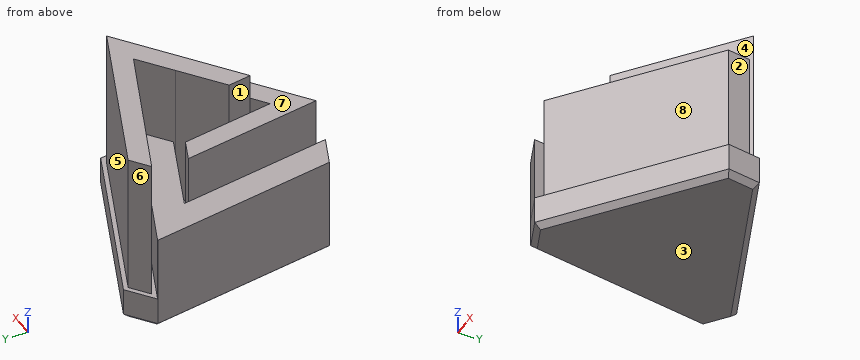
```python
from build123d import *

# Parameters (mm, degrees)
F1_DEPTH = 30
F5_DEPTH = 60
F6_DEPTH = 100
F7_DEPTH = 130
F8_SIZE  = 5


with BuildPart() as f1:
    # F0 (on Top) → F1 (new body)
    with BuildSketch(Plane.XY):
        Polygon((-39.487894, -75.850017), (94.227236, 28.575137), (90.058191, 58.284042), (-67.23421, 121.872165), (-90.878354, 103.407213), (-67.301084, -64.606063), align=None)
    extrude(amount=F1_DEPTH)

    # F2 (on face) → F5 (join)
    with BuildSketch(Plane.XY.offset(30)):
        Polygon((14.600857, 32.81471), (37.999574, 51.148787), (-90.714814, 103.534931), (-90.878354, 103.407213), (-67.301084, -64.606063), (-40.06353, -75.617306), (-59.289651, 62.461207), (-30.906815, 51.073389), align=None)
    extrude(amount=F5_DEPTH)

    # F4 (on face) → F6 (join)
    with BuildSketch(Plane.XY.offset(30)):
        Polygon((87.029812, 51.080902), (-23.003388, -34.692019), (-28.099764, 1.909229), (-34.548747, 48.224661), (-54.376458, 56.179975), (-36.972718, -68.81053), (89.945114, 30.306257), align=None)
    extrude(amount=F6_DEPTH)

    # F3 (on face) → F7 (join)
    with BuildSketch(Plane.XY.offset(30)):
        Polygon((17.067929, 29.66613), (-19.8587, 0.732249), (-16.991157, -19.861924), (81.935531, 57.253266), (-66.592344, 117.29818), (-82.807181, 104.635163), (45.895328, 52.253855), align=None)
    extrude(amount=F7_DEPTH)

    # F8
    f8_edges = [f1.edges().sort_by_distance(p)[0] for p in [
        (11.41199, 90.078103, 0),
        (92.142713, 43.429589, 0),
        (27.369671, -23.63744, 0),
        (-79.056282, 112.639689, 0),
        (-79.089719, 19.400575, 0),
        (-53.394489, -70.22804, 0),
    ]]
    chamfer(f8_edges, length=F8_SIZE)


solid = f1.part
```
Read the model definition and answer for the solid it produces. Units are mm, in the model's axes. Face numbers are marked on the shaded views. A direction names the side the tool comes from. Coordinates: 2 decimals unless noted, no trailing zeros. Write each loop counter-clockwise with the first axis right and the second up, starting at its lowest first coordinate (ties: lowest second). Pieces come first, ordered by that corner, then holes. Notation, with made-up numbers: (-4, -8.5) -> (1, -8.5) arc R23 ccw to (1, 29.5) -> close; hole circle Ø5 at (30.25, 0). An arc over 180 degrees is marked (long way). Write item = value, one per line.
(1) Which of the six approach directions +Z, -Z, +X, -X, +Y, -Y give full straight-line access (tool end or side, diameter ignored) to the marked faces 4, 5, 6, 7 and 8?
From the geometry:
face_4 = +Z
face_5 = +Z, +X, +Y
face_6 = +Z, -X, +Y
face_7 = +Z, -Y
face_8 = +Z, +X, -Y
(2) For a pull along X with two mould halves and no side action, classify the marked faces 1, 2 and 3 as +X half, -X half, draft (parallel to the pull), parting line (faces both ways), or undercut.
From the geometry:
face_1 = undercut
face_2 = +X half
face_3 = draft
(3) Section B-B on z = 48 is taken. Write down the section's boundary in (x, y), plus the area to 3 significant figures.
From the geometry:
outline = (-90.88, 103.41) -> (-67.3, -64.61) -> (-40.06, -75.62) -> (-59.29, 62.46) -> (14.6, 32.81) -> (38, 51.15) -> (-90.71, 103.53) -> close; (-82.81, 104.64) -> (45.9, 52.25) -> (-19.86, 0.73) -> (-16.99, -19.86) -> (81.94, 57.25) -> (-66.59, 117.3) -> close; (-54.38, 56.18) -> (-36.97, -68.81) -> (89.95, 30.31) -> (87.03, 51.08) -> (-23, -34.69) -> (-34.55, 48.22) -> close
area = 16,100 mm2
(4) Given pin 1 Ø1.5 at (x, z) = (49, 69) entering from -Y; pin 2 Ø6 at (y, z) = (36, 133.5) entering from -X; pin 3 Ø12 at (y, z) = (-13.5, 109.5) entering from -X, each flat-ended and moving along its own axis, determine where each tip first touches the part or whether it passes through.
From the geometry:
pin_1 = -2.26
pin_2 = 21.32
pin_3 = -45.51
(5) Section C-C on x = 2.5 is taken. Write down the section's boundary in (y, z).
From the geometry:
outline = (-43.06, 5) -> (-36.72, 0) -> (88.29, 0) -> (93.68, 5) -> (93.68, 30) -> (89.37, 30) -> (89.37, 160) -> (69.92, 160) -> (69.92, 30) -> (65.6, 30) -> (65.6, 90) -> (37.67, 90) -> (37.67, 30) -> (18.25, 30) -> (18.25, 160) -> (-4.67, 160) -> (-4.67, 30) -> (-14.81, 30) -> (-14.81, 130) -> (-37.98, 130) -> (-37.98, 30) -> (-43.06, 30) -> close
(6) Section A-A on z = 112.5 is taken. Write down the section's boundary in (x, y).
From the geometry:
outline = (-82.81, 104.64) -> (45.9, 52.25) -> (-19.86, 0.73) -> (-16.99, -19.86) -> (81.94, 57.25) -> (-66.59, 117.3) -> close; (-54.38, 56.18) -> (-36.97, -68.81) -> (89.95, 30.31) -> (87.03, 51.08) -> (-23, -34.69) -> (-34.55, 48.22) -> close
(7) Straight lines are drawn through the part: L1, parallel to X at y = 18.5, z = 111.5; L2, parallel to Y at x = 10, z = 111; L3, parallel to X at y = -18, z = 52. For each, find the intervals that lie inside material, in ascending order. Write a range as from..to.
From the geometry:
L1 = -49.13..-30.41, 2.82..32.22, 45.23..74.83
L2 = -32.13..-8.97, 1.18..24.13, 66.86..86.33
L3 = -73.84..-48.09, -44.05..-25.33, -17.25..-14.6, -1.59..28.09
(8) Section D-D on y = 98 is taken. Write down the section's boundary in (x, z).
From the geometry:
outline = (-90.12, 5) -> (-85.07, 0) -> (-21.52, 0) -> (-8.18, 5) -> (-8.18, 30) -> (-18.86, 30) -> (-18.86, 160) -> (-66.5, 160) -> (-66.5, 30) -> (-77.12, 30) -> (-77.12, 90) -> (-90.12, 90) -> close
